Build history of the part. All positions in model axes, mm. Give positions to 0.01 mm unless a question says otherwise; leave off trailing zeros. Order: outer loops, then holes, each group sorted by start corner. A loop starts at its lowest first (then second) coordinate and runs counter-clockwise, first axis right, second up. Notation, with made-up numbers: (66.5, -5) - (99.5, -5) arc R25 ccw to (99.5, 10) - close; hole circle Ø6 at (-36.75, 2). An arc over 180 degrees is marked (long way). Use a Markdown table: item, result.
from build123d import *

# Parameters (mm, degrees)
EXTRUDE_1_DEPTH     = 8.5
SKETCH_2_R          = 2.1
CUT_EXTRUDE_1_DEPTH = 10


with BuildPart() as part:
    # 草图1 → 凸台-拉伸1 (new body)
    with BuildSketch(Plane.XY):
        with BuildLine():
            Line((-119.733036377, -8), (-109.733036377, -8))
            Line((-109.733036377, -8), (-109.733036377, -48.566045006))
            ThreePointArc((-109.733036377, -48.566045006), (0, -120), (109.733036377, -48.566045006))
            Line((109.733036377, -48.566045006), (109.733036377, -8))
            Line((109.733036377, -8), (119.733036377, -8))
            ThreePointArc((119.733036377, -8), (119.873837168, -5.50119648), (119.962494139, -3))
            Line((119.962494139, -3), (100.955435713, -3))
            ThreePointArc((100.955435713, -3), (99.617551315, -16.653632338), (96.441692229, -30))
            Line((96.441692229, -30), (91.192104921, -30))
            ThreePointArc((91.192104921, -30), (0, -96), (-91.192104921, -30))
            Line((-91.192104921, -30), (-96.441692229, -30))
            ThreePointArc((-96.441692229, -30), (-99.617551315, -16.653632338), (-100.955435713, -3))
            Line((-100.955435713, -3), (-119.962494139, -3))
            ThreePointArc((-119.962494139, -3), (-119.873837168, -5.50119648), (-119.733036377, -8))
        make_face()
    extrude(amount=EXTRUDE_1_DEPTH)

    # 草图2 → 切除-拉伸1 (cut)
    with BuildSketch(Plane(origin=(0, -3, 0), x_dir=(1, 0, 0), z_dir=(0, 1, 0))):
        with Locations(Location((-114.962494139, -4.25, 0), (0, 0, 270))):
            Circle(SKETCH_2_R)
        with Locations(Location((114.962494139, -4.25, 0), (0, 0, 270))):
            Circle(SKETCH_2_R)
    extrude(amount=-CUT_EXTRUDE_1_DEPTH, mode=Mode.SUBTRACT)


solid = part.part
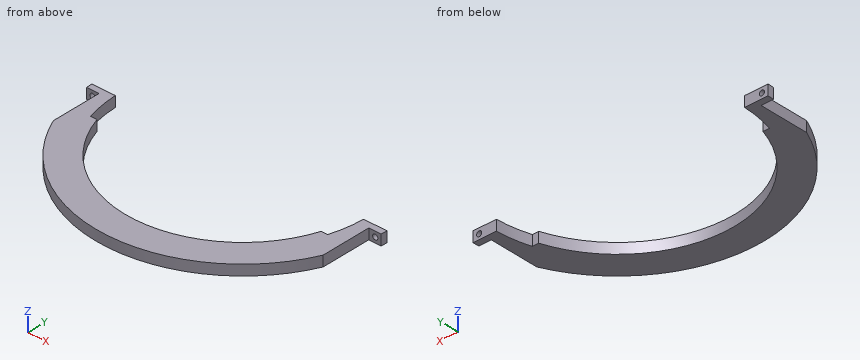
1) Slice it at D-D (x = 79). Write the cut outline in (y, z), and give its area (3 significant figures).
Computed:
| item | result |
|---|---|
| outline | (-90.33, 0) - (-54.54, 0) - (-54.54, 8.5) - (-90.33, 8.5) - close |
| area | 304 mm² |
2) Slice it at B-B (y = -54). Write the cut outline in (x, z), and give its area (3 significant figures).
Computed:
| item | result |
|---|---|
| outline | (-107.16, 0) - (-79.37, 0) - (-79.37, 8.5) - (-107.16, 8.5) - close; (79.37, 0) - (107.16, 0) - (107.16, 8.5) - (79.37, 8.5) - close |
| area | 472 mm² |
3) Pin check, flat tips, straight feed: P1, Ø1, axis at y = -71, z = 2, coming from the +X side; P2, Ø4, axis at x = 93.5, z = 6, coming from the +Y side; P3, Ø2.5, axis at x = -114, z = 5, coming from the -Y side. Stop position of each tip, or through.
Computed:
| item | result |
|---|---|
| P1 | stops at x = 97.11 |
| P2 | stops at y = -30 |
| P3 | stops at y = -8 |
4) Wall check: line 1 (X direction, y = -4.05, z = 4.25); line 2 (X direction, y = -5.7, z = 4.25); line 3 (Y direction, x = -1.5, z = 8). Give the ranges that are in metal, low to high. Write a range as from..to.
Computed:
| item | result |
|---|---|
| line 1 | x = -119.93..-117.06, -112.86..-100.92, 100.92..112.86, 117.06..119.93 |
| line 2 | x = -119.86..-117.06, -112.86..-100.84, 100.84..112.86, 117.06..119.86 |
| line 3 | y = -119.99..-95.99 |
5) Slice it at C-C (y = -25). Write the cut outline in (x, z).
Computed:
| item | result |
|---|---|
| outline | (-109.73, 0) - (-97.86, 0) - (-97.86, 8.5) - (-109.73, 8.5) - close; (97.86, 0) - (109.73, 0) - (109.73, 8.5) - (97.86, 8.5) - close |
6) Slice it at A-A (z = 4.25). Write the cut outline in (x, y), and give its area (3 significant figures).
Computed:
| item | result |
|---|---|
| outline | (-119.96, -3) arc R120 ccw to (-119.73, -8) - (-117.06, -8) - (-117.06, -3) - close; (-112.86, -8) - (-109.73, -8) - (-109.73, -48.57) arc R120 ccw to (109.73, -48.57) - (109.73, -8) - (112.86, -8) - (112.86, -3) - (100.96, -3) arc R101 cw to (96.44, -30) - (91.19, -30) arc R96 cw to (-91.19, -30) - (-96.44, -30) arc R101 cw to (-100.96, -3) - (-112.86, -3) - close; (117.06, -8) - (119.73, -8) arc R120 ccw to (119.96, -3) - (117.06, -3) - close |
| area | 7,170 mm² |
